Can you work these out from the model? Positions are in its coordinate system, mm. Face numbers are marked on the shaded views. A direction names the side the tool comes from. Give positions to 0.01 mm unless a question says otherwise; leave off trailing zeros. Write item = value, one per line.
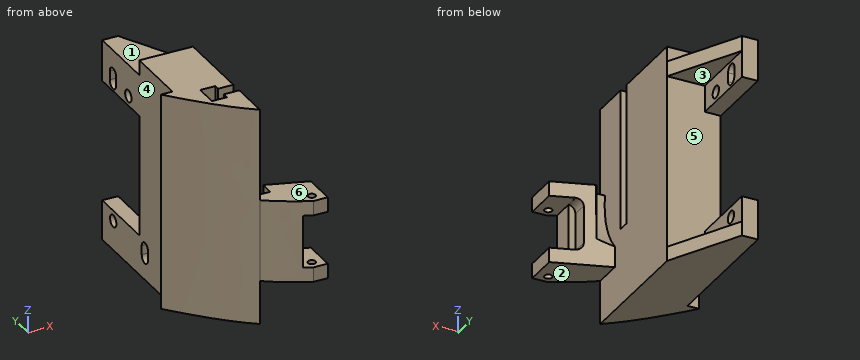
from build123d import *

# Parameters (mm, degrees)
BOSS_EXTRUDE1_DEPTH = 73.406
SKETCH2_W           = 5.08
SKETCH2_H           = 23.996252619
SKETCH2_W_2         = 40.894
CUT_EXTRUDE1_DEPTH  = 112.686247001
SKETCH3_W           = 58.42
SKETCH3_H           = 23.996252619
CUT_EXTRUDE2_DEPTH  = 12.7
SKETCH4_R           = 2.032
CUT_EXTRUDE3_DEPTH  = 114.950293405
SKETCH5_W           = 30.988
SKETCH5_H           = 17.263986836
SKETCH5_W_2         = 14.732
CUT_EXTRUDE4_DEPTH  = 18.796
CUT_EXTRUDE5_DEPTH  = 47.498
SKETCH7_W           = 7.62
SKETCH7_H           = 17.78
CUT_EXTRUDE6_DEPTH  = 22.098
CUT_EXTRUDE7_DEPTH  = 42.164
SKETCH9_R           = 1.27
CUT_EXTRUDE8_DEPTH  = 777.033475109
CUT_EXTRUDE9_DEPTH  = 5.08
FILLET1_R           = 0.254


with BuildPart() as part:
    # Sketch1 → Boss-Extrude1 (new body)
    with BuildSketch(Plane.XY):
        with BuildLine():
            Line((-748.665, -64.002429831), (-748.665, -30.220429831))
            Line((-748.665, -30.220429831), (-761.365, -6.224177212))
            Line((-761.365, -6.224177212), (-766.699, -6.224177212))
            Line((-766.699, -6.224177212), (-766.699, -51.658164167))
            Line((-766.699, -51.658164167), (-770.600050032, -51.658164167))
            add(Edge.make_bspline(
                [(-770.600050032, -51.658164167), (-769.474110637, -53.020450544), (-766.896191207, -56.054888677), (-762.734517182, -60.657959907), (-758.1103328, -65.445789554), (-753.453331209, -69.75760173), (-750.223005304, -72.311764833), (-748.665, -73.440199402)],
                knots=[0.071886948, 0.071886948, 0.071886948, 0.071886948, 0.078125, 0.0859375, 0.09375, 0.1015625, 0.108408754, 0.108408754, 0.108408754, 0.108408754], degree=3))
            Line((-748.665, -73.440199402), (-748.665, -64.002429831))
        make_face()
        with BuildLine():
            Line((-729.869, -70.265959359), (-748.665, -64.002429831))
            Line((-748.665, -64.002429831), (-748.665, -73.440199402))
            add(Edge.make_bspline(
                [(-748.665, -73.440199402), (-748.445110963, -73.599460985), (-744.652568783, -76.312065429), (-739.987854595, -78.967573397), (-735.357324532, -81.008335743), (-734.751026936, -81.266416667)],
                knots=[0.108408754, 0.108408754, 0.108408754, 0.108408754, 0.109375, 0.125, 0.127339677, 0.127339677, 0.127339677, 0.127339677], degree=3))
            Line((-734.751026936, -81.266416667), (-729.869, -81.266416667))
            Line((-729.869, -81.266416667), (-729.869, -70.265959359))
        make_face()
    extrude(amount=BOSS_EXTRUDE1_DEPTH)

    # Sketch2 → Cut-Extrude1 (cut, through all)
    with BuildSketch(Plane(origin=(-748.665, 0, 0), x_dir=(0, 0, -1), z_dir=(1, 0, 0))):
        with Locations((-70.866, -18.222303522)):
            Rectangle(SKETCH2_W, SKETCH2_H)
        with Locations((-33.909, -18.222303522)):
            Rectangle(SKETCH2_W_2, SKETCH2_H)
    extrude(amount=-CUT_EXTRUDE1_DEPTH, mode=Mode.SUBTRACT)

    # Sketch3 → Cut-Extrude2 (cut)
    with BuildSketch(Plane(origin=(-748.665, 0, 0), x_dir=(0, 0, -1), z_dir=(1, 0, 0))):
        with Locations((-34.036, -18.222303522)):
            Rectangle(SKETCH3_W, SKETCH3_H)
    extrude(amount=-CUT_EXTRUDE2_DEPTH, mode=Mode.SUBTRACT)

    # Sketch4 → Cut-Extrude3 (cut, through all)
    with BuildSketch(Plane(origin=(-761.365, 0, 0), x_dir=(0, 0, -1), z_dir=(1, 0, 0))):
        with Locations((-57.610523574, -23.108429831)):
            Circle(SKETCH4_R)
        with Locations((-9.906, -13.336177212)):
            Circle(SKETCH4_R)
        with BuildLine():
            Line((-60.198, -11.101802223), (-57.15, -11.101802223))
            ThreePointArc((-57.15, -11.101802223), (-55.118, -13.133802223), (-57.15, -15.165802223))
            Line((-57.15, -15.165802223), (-60.198, -15.165802223))
            ThreePointArc((-60.198, -15.165802223), (-62.23, -13.133802223), (-60.198, -11.101802223))
        make_face()
        with BuildLine():
            Line((-10.668, -31.774706288), (-7.62, -31.774706288))
            ThreePointArc((-7.62, -31.774706288), (-5.588, -33.806706288), (-7.62, -35.838706288))
            Line((-7.62, -35.838706288), (-10.668, -35.838706288))
            ThreePointArc((-10.668, -35.838706288), (-12.7, -33.806706288), (-10.668, -31.774706288))
        make_face()
    extrude(amount=-CUT_EXTRUDE3_DEPTH, mode=Mode.SUBTRACT)

    # Sketch5 → Cut-Extrude4 (cut)
    with BuildSketch(Plane(origin=(-729.869, 0, 0), x_dir=(0, 0, -1), z_dir=(1, 0, 0))):
        with Locations((-57.912, -72.634423249)):
            Rectangle(SKETCH5_W, SKETCH5_H)
        with Locations((-7.366, -72.634423249)):
            Rectangle(SKETCH5_W_2, SKETCH5_H)
    extrude(amount=-CUT_EXTRUDE4_DEPTH, mode=Mode.SUBTRACT)

    # Sketch6 → Cut-Extrude5 (cut)
    with BuildSketch(Plane.XY.offset(73.406)):
        Polygon((-748.665, -56.374416667), (-748.665, -60.184416667), (-753.836367364, -60.184416667), (-753.836367364, -62.216416667), (-758.916367364, -62.216416667), (-758.916367364, -54.596416667), (-753.836367364, -54.596416667), (-753.836367364, -56.374416667), align=None)
    extrude(amount=-CUT_EXTRUDE5_DEPTH, mode=Mode.SUBTRACT)

    # Sketch7 → Cut-Extrude6 (cut)
    with BuildSketch(Plane.XZ.offset(81.266416667)):
        with Locations((-733.679, 28.575)):
            Rectangle(SKETCH7_W, SKETCH7_H)
    extrude(amount=-CUT_EXTRUDE6_DEPTH, mode=Mode.SUBTRACT)

    # Sketch8 → Cut-Extrude7 (cut)
    with BuildSketch(Plane(origin=(0, -30.220429831, 0), x_dir=(1, 0, 0), z_dir=(0, 1, 0))):
        with BuildLine():
            Line((-729.869, -37.465), (-737.235, -37.465))
            ThreePointArc((-737.235, -37.465), (-739.031051224, -36.721051224), (-739.775, -34.925))
            Line((-739.775, -34.925), (-739.775, -22.225))
            ThreePointArc((-739.775, -22.225), (-739.031051224, -20.428948776), (-737.235, -19.685))
            Line((-737.235, -19.685), (-729.869, -19.685))
            Line((-729.869, -19.685), (-729.869, -37.465))
        make_face()
    extrude(amount=-CUT_EXTRUDE7_DEPTH, mode=Mode.SUBTRACT)

    # Sketch9 → Cut-Extrude8 (cut, through all)
    with BuildSketch(Plane.XY.offset(42.418)):
        with Locations((-733.679, -78.218416667)):
            Circle(SKETCH9_R)
    extrude(amount=-CUT_EXTRUDE8_DEPTH, mode=Mode.SUBTRACT)

    # Sketch12 → Cut-Extrude9 (cut)
    with BuildSketch(Plane(origin=(-748.665, 0, 0), x_dir=(0, 0, -1), z_dir=(1, 0, 0))):
        with BuildLine():
            Line((-42.418, -64.002429831), (-21.844, -64.002429831))
            ThreePointArc((-21.844, -64.002429831), (-31.440091509, -69.415973341), (-42.418, -70.352429831))
            Line((-42.418, -70.352429831), (-42.418, -64.002429831))
        make_face()
    extrude(amount=CUT_EXTRUDE9_DEPTH, mode=Mode.SUBTRACT)

    # Fillet1
    fillet1_edges = [part.edges().sort_by_distance(p)[0] for p in [
        (-743.585, -65.69527565, 33.18708051),
        (-746.106672699, -64.854960082, 22.851173008),
    ]]
    fillet(fillet1_edges, radius=FILLET1_R)


solid = part.part
Q1. Imagine slicing it at A-A, the plane x = -763.5. Give the number of separate pieces and of enclosed holes in the cut face, then the cut area to 3 significant figures.
Output:
separate_pieces = 1
enclosed_holes = 4
area = 2,750 mm2
Q2. We'd pull the mould along Z, two halves only. Please class the marked faces 4, 5 and 6: released by +Z, released by -Z, zero draft, split by the parting line, or undercut.
Output:
face_4 = zero draft
face_5 = undercut
face_6 = released by +Z
Q3. Which directions (+Z, -Z, +X, -X, +Y, -Y) give clear straight access to the entire face, cutting with the end or side of a thin tool? Please do the marked faces 1, 2 and 3.
Output:
face_1 = +Z, +X, -X, +Y
face_2 = -Z, +X, +Y, -Y
face_3 = +X, +Y
Q4. For pin 1 (13 mm diameter, centred on y = -46, z = 46, fed in from +X) (3 decimals); pin 2 (9 mm diameter, centred on x = -758, y = -12.5, fed in from +Z); pin 3 (4.5 mm diameter, centred on y = -15.5, z = 7.5, fed in from +X) (3 decimals), each with a flat end and sliding along its axis, tell me the tip position at first contact or that it passes through.
Output:
pin_1 = -748.665
pin_2 = 68.33
pin_3 = -761.365
Q5. I need wall thicknesses on L1, parallel to Z at x = -736, y = -76.5 (3 decimals); L2, parallel to Z at x = -757, y = -22.5; L3, parallel to Y at x = -764, z = 59. Which ranges of each line are inside material? Lowest first, please.
Output:
L1 = 14.732 to 19.685, 37.465 to 42.418
L2 = 0 to 4.83, 63.25 to 68.33
L3 = -59.24 to -24.59, -21.63 to -15.17, -11.1 to -6.22
